```python
from build123d import *

# Parameters (mm, degrees)
PAD001_DEPTH = 116.4
THICKNESS_T  = 1


with BuildPart() as part:
    # Sketch001 → Pad001 (new body)
    with BuildSketch(Plane.XZ):
        Polygon((0, 67.8), (-39.144348, 90.4), (-78.288697, 67.8), (-78.288697, 22.6), (-39.144348, 0), (0, 22.6), (39.144348, 0), (78.288697, 22.6), (78.288697, 67.8), (39.144348, 90.4), align=None)
    extrude(amount=PAD001_DEPTH)

    # Thickness
    thickness_openings = [part.faces().sort_by_distance(p)[0] for p in [
        (58.716522, -58.2, 79.1),
        (-19.572174, -58.2, 79.1),
        (19.572174, -58.2, 79.1),
        (-58.716522, -58.2, 79.1),
    ]]
    offset(amount=THICKNESS_T, openings=thickness_openings)


solid = part.part
```
Here's how the part is built. I have some questions about the finished solid (model axes, mm). A direction names the side the tool comes from. Round coordinates to 2 decimals unless told otherwise and drop trailing zeros. Order: outer loops, then holes, each group sorted by start corner. A loop starts at its lowest first (then second) coordinate and runs counter-clockwise, first axis right, second up. Notation, with made-up numbers: M -12,4.5 L 25,4.5 A4 cw 25,9.5 Z; hole C -35.75,86.5 d10. An arc over 180 degrees is marked long. Use CSV: the item, a comma, the result in double quotes.
1) I need wall thicknesses on line 1 along Y through (x, z) = (-19.5, 78.5); line 2 along X through (y, z) = (-49.5, 32); line 3 along X through (y, z) = (-80.5, 4). Which ranges of each line are inside material? Lowest first, please. Write a range as [from, to].
Taken from the geometry:
line 1,"[-117.4, -116.4], [0, 1]"
line 2,"[-79.29, -78.29], [78.29, 79.29]"
line 3,"[-48.07, -46.07], [-32.22, -30.22], [30.22, 32.22], [46.07, 48.07]"
2) I want a section at A-A (z = 49.5). List the corners of the cut face in (x, y) for me.
Taken from the geometry:
outline,"M -79.29,-116.4 A1 ccw -78.29,-117.4 L 78.29,-117.4 A1 ccw 79.29,-116.4 L 79.29,0 A1 ccw 78.29,1 L -78.29,1 A1 ccw -79.29,0 Z; hole M -78.29,-116.4 L 78.29,-116.4 L 78.29,0 L -78.29,0 Z"
3) I want a section at C-C (y = -39.5). List the corners of the cut face in (x, z) for me.
Taken from the geometry:
outline,"M -79.29,22.6 A1 ccw -78.79,21.73 L -39.64,-0.87 A1 ccw -38.64,-0.87 L 0,21.45 L 38.64,-0.87 A1 ccw 39.64,-0.87 L 78.79,21.73 A1 ccw 79.29,22.6 L 79.29,67.22 L 78.29,67.8 L 78.29,22.6 L 39.14,0 L 0,22.6 L -39.14,0 L -78.29,22.6 L -78.29,67.8 L -79.29,67.22 Z"
4) On a 3-axis mill with a long thin cutter (end or side, diameter ignored), from which of +Z, -Z, +X, -X, +Y, -Y can I reach the whole of each face in a straight line? I mean faces 1 (the flat face through (19.052, -57.385, 10.446)), 2 (the flat face through (78.289, -57, 45)), 3 (the cylindrical face through (-18.94, -117.1, 10.84)), 4 (the cylindrical face through (-18.94, 0.7, 10.84)). Say none if no direction works.
Taken from the geometry:
face 1,"-Z, +Y, -Y"
face 2,"+Z"
face 3,"-Z, -Y"
face 4,"-Z, +Y"
5) I want a section at B-B (z = 74.5). List the corners of the cut face in (x, y) for me, then the cut area to 3 significant figures.
Taken from the geometry:
outline,"M -66.68,-117.4 L -11.6,-117.4 L -11.6,-116.4 L -66.68,-116.4 Z; M -66.68,0 L -11.6,0 L -11.6,1 L -66.68,1 Z; M 11.6,-117.4 L 66.68,-117.4 L 66.68,-116.4 L 11.6,-116.4 Z; M 11.6,0 L 66.68,0 L 66.68,1 L 11.6,1 Z"
area,"220 mm^2"
6) I'm going to push flat-ended pins straight in: P1, Ø6, axis at x = -16, y = -90, coming from the +Z side; P2, Ø12, axis at x = 28, y = -74.5, coming from the +Z side; P3, Ø8, axis at x = -59.5, y = -53, coming from the +Z side. Where does each tip first touch, or does it pass through?
Taken from the geometry:
P1,"z = 15.09"
P2,"z = 9.9"
P3,"z = 14.06"
7) If we mould it in two halves opening along Y, with no side actions, what happens to faces 5 (the flat face through (58.44, -57.39, 11.14)), 6 (the cylindrical face through (19.49, -117.1, 10.52)), 7 (the flat face through (19.85, 0.51, 79.26))? For each: pulls with the +Y half, pulls with the -Y half, needs draft (parallel to the pull), parting line crosses it, or undercut.
Taken from the geometry:
face 5,"undercut"
face 6,"pulls with the -Y half"
face 7,"needs draft"
8) I want a section at D-D (z = 8.5). Count the separate pieces of the cut face and the enclosed holes in it, then the cut area to 3 significant figures.
Taken from the geometry:
separate pieces,"2"
enclosed holes,"2"
area,"1,060 mm^2"
